```python
from build123d import *

# Parameters (mm, degrees)
SKETCH_1_R               = 40
EXTRUDE_1_DEPTH          = 50
CUT_EXTRUDE_1_DEPTH      = 15
CUT_EXTRUDE_1_DEPTH_BACK = 16
SKETCH_2_OUTSIDE_W       = 106.738
SKETCH_2_OUTSIDE_H       = 106.738
SKETCH_2_OUTSIDE_R       = 30
FILLET_1_R               = 10
FILLET_2_R               = 10
CUT_EXTRUDE_2_DEPTH      = 62.846584384
CUT_EXTRUDE_2_DEPTH_BACK = 62.846584384
SKETCH_3_R               = 10


with BuildPart() as part:
    # 草图1 → 凸台-拉伸1 (new body)
    with BuildSketch(Plane.XY):
        Circle(SKETCH_1_R)
    extrude(amount=EXTRUDE_1_DEPTH)

    # 草图2 outside → 切除-拉伸1 (cut, two sides: drawn at the far end of the back side and taken through both)
    with BuildSketch(Plane.XY.offset(25).offset(-CUT_EXTRUDE_1_DEPTH_BACK)):
        Rectangle(SKETCH_2_OUTSIDE_W, SKETCH_2_OUTSIDE_H)
        Circle(SKETCH_2_OUTSIDE_R, mode=Mode.SUBTRACT)
    extrude(amount=CUT_EXTRUDE_1_DEPTH + CUT_EXTRUDE_1_DEPTH_BACK, mode=Mode.SUBTRACT)

    # 圆角1
    fillet_1_edges = [part.edges().sort_by_distance(p)[0] for p in [
        (-30, 0, 40),
    ]]
    fillet(fillet_1_edges, radius=FILLET_1_R - 0.0001)  # a hair under: the kernel refuses the full size

    # 圆角2
    fillet_2_edges = [part.edges().sort_by_distance(p)[0] for p in [
        (-30, 0, 9),
    ]]
    fillet(fillet_2_edges, radius=FILLET_2_R - 0.0001)  # a hair under: the kernel refuses the full size

    # 草图3 → 切除-拉伸2 (cut, two sides: drawn at the far end of the back side and taken through both)
    with BuildSketch(Plane.XY.offset(25).offset(-CUT_EXTRUDE_2_DEPTH_BACK)):
        Circle(SKETCH_3_R)
    extrude(amount=CUT_EXTRUDE_2_DEPTH + CUT_EXTRUDE_2_DEPTH_BACK, mode=Mode.SUBTRACT)


solid = part.part
```
Can you work these out from the model? Positions are in its coordinate system, mm. Round coordinates to 2 decimals unless told otherwise and drop trailing zeros. Loops run counter-clockwise (first coordinate to the right, second up) from the corner with the lowest first, then second, coordinate; pieces in that order, holes last. Notation, with made-up numbers: M 80.5,82 L 108.5,82 A28 ccw 108.5,104 Z; hole C -18,36 d4. An arc over 180 degrees is marked long. Answer in a Markdown table with one row per item.
1. Thinking about a two-plate mould opening in Z: for faces 1 (the face through (-2.17, -9.76, 24.65)), 2 (the face through (-29.97, 1.32, 24.42)), 3 (the face through (8, -8, 50)), which applies, pulls with the +Z half, pulls with the -Z half, needs draft (parallel to the pull), parting line crosses it, or undercut?
Established:
| item | result |
|---|---|
| face 1 | needs draft |
| face 2 | undercut |
| face 3 | pulls with the +Z half |
2. Please list where these lines run through material, in increasing order: line 1 (Y direction, x = 0, z = 23); line 2 (Y direction, x = 0, z = 34); line 3 (X direction, y = 8, z = 25.5). Write a range as from..to.
Established:
| item | result |
|---|---|
| line 1 | -30..-10, 10..30 |
| line 2 | -30.83..-10, 10..30.83 |
| line 3 | -28.91..-6, 6..28.91 |
3. I'm going to push flat-ended pins straight in: pin 1 Ø10 at (y, z) = (7, 36.5) entering from +X; pin 2 Ø6 at (x, z) = (12.5, 20) entering from -Y; pin 3 Ø6 at (y, z) = (11, 36) entering from -X. Where does each tip first touch, or does it pass through?
Established:
| item | result |
|---|---|
| pin 1 | x = 39.85 |
| pin 2 | y = -28.46 |
| pin 3 | x = -33.97 |
4. If we section it at C-C, the plane z = 8: Please give me the cut outline in (x, y).
Established:
| item | result |
|---|---|
| outline | C 0,0 d80; hole C 0,0 d20 |
